Check sheet for the modelled part. Datum: model origin and axes. Units: mm. Round coordinates to 2 decimals unless told otherwise and drop trailing zeros. Write each loop counter-clockwise with the first axis right and the second up, starting at its lowest first coordinate (ties: lowest second). Pieces come first, ordered by that corner, then holes. Notation, with made-up numbers: (-31, 81) -> (-2, 81) arc R17 ccw to (-2, 114) -> close; hole circle Ø8 at (-5, 9.25). An arc over 180 degrees is marked (long way). Answer as a JSON object with one key per item and string values. Group by question number.
```python
from build123d import *

# Parameters (mm, degrees)
F0_R     = 48.5
F1_DEPTH = 5


with BuildPart() as f1:
    # F0 (on Front) → F1 (new body)
    with BuildSketch(Plane.XZ):
        Circle(F0_R)
        with BuildLine():
            ThreePointArc((-20.961748, -27.960622), (-25.727517, -29.017168), (-21.854779, -26.045511))
            ThreePointArc((-21.854779, -26.045511), (-21.195978, -26.904077), (-20.961748, -27.960622))
        make_face(mode=Mode.SUBTRACT)
        with BuildLine():
            ThreePointArc((34.109927, -18.25), (30.96288, -20.664815), (29.444864, -17))
            ThreePointArc((29.444864, -17), (32.256975, -15.835185), (34.109927, -18.25))
        make_face(mode=Mode.SUBTRACT)
        with BuildLine():
            ThreePointArc((-15.748296, -18.768089), (-22.204541, -10.354147), (-24.5, 0))
            ThreePointArc((-24.5, 0), (-14.052623, 20.069225), (8.379494, 23.022469))
            ThreePointArc((8.379494, 23.022469), (20.069225, 14.052623), (24.5, 0))
            ThreePointArc((24.5, 0), (23.665183, -6.341067), (21.217622, -12.25))
            ThreePointArc((21.217622, -12.25), (4.25438, -24.12779), (-15.748296, -18.768089))
        make_face(mode=Mode.SUBTRACT)
        with BuildLine():
            ThreePointArc((14.983735, 34.298781), (13.917676, 32.250901), (11.628685, 31.949549))
            ThreePointArc((11.628685, 31.949549), (11.049794, 36.346661), (14.983735, 34.298781))
        make_face(mode=Mode.SUBTRACT)
    extrude(amount=F1_DEPTH)


solid = f1.part
```
(1) Section check C-C on y = -3.15. Record the cut outline in (x, z).
(2) Release check for a two-part mould opening along Z. For faces 1 (the cylindrical face through (23.69, -2.46, -6.25)), 2 (the flat face through (-22.2, 0, 11.5)), 3 (the cylindrical face through (22.38, -2.465, -43.028)) record: pulls with the +Z half, pulls with the -Z half, needs draft (parallel to the pull), parting line crosses it, or undercut.
(3) Go/stop test with a flat-tipped pin: pin 1 Ø3 at (x, z) = (31.61, -18.25) entering from +Y. Record where the tip stops, or that it passes through.
(4) Section check A-A on x = 0. Record the cut outline in (y, z), then the cut area to 3 significant figures.
(5) Scan lines: line 1 along X through (y, z) = (-0.4, 0.5); line 2 along Z through (x, y) = (11, -4.55); line 3 along Z through (x, y) = (9, -4.3). Record each from-to range of solid material in increasing order.
(6) Section check B-B on z = 13.5. Record the cut outline in (x, y).
Data:
{
 "1": {"outline": "circle Ø97 at (0, 0); hole (-24.5, 0) arc R24.5 ccw to (-15.75, -18.77) arc R24.5 ccw to (21.22, -12.25) arc R24.5 ccw to (24.5, 0) arc R24.5 ccw to start; hole (-21.85, -26.05) arc R2.5 ccw (long way) to (-20.96, -27.96) arc R2.5 ccw to start; hole circle Ø5 at (12.48, 34.3); hole (29.44, -17) arc R2.5 ccw (long way) to (34.11, -18.25) arc R2.5 ccw to start"},
 "2": {"face 1": "undercut", "face 2": "needs draft", "face 3": "parting line crosses it"},
 "3": {"pin 1": "passes through"},
 "4": {"outline": "(-5, -48.5) -> (0, -48.5) -> (0, -24.5) -> (-5, -24.5) -> close; (-5, 24.5) -> (0, 24.5) -> (0, 48.5) -> (-5, 48.5) -> close", "area": "240 mm²"},
 "5": {"line 1": "x = -48.5 to -24.49, 24.49 to 48.5", "line 2": "z = -47.24 to -21.89, 21.89 to 32.29, 36.31 to 47.24", "line 3": "z = -47.66 to -22.79, 22.79 to 47.66"},
 "6": {"outline": "(-46.58, -5) -> (-20.45, -5) -> (-20.45, 0) -> (-46.58, 0) -> close; (20.45, -5) -> (46.58, -5) -> (46.58, 0) -> (20.45, 0) -> close"}
}
